For this review, use the dimensioned drawing (mm, ordinates from the lowest corner) and the shaded views. A direction names the side the tool comes from. Round coordinates to 2 decimals unless told otherwise and drop trailing zeros. Loops run counter-clockwise (first coordinate to the right, second up) from the corner with the lowest first, then second, coordinate; pieces in that order, holes last. Notation, with made-up numbers: M 4,55 L 48,55 A32 cw 48,91 Z; hole C 37,46.5 d7. An arc over 180 degrees is marked long. Answer as a JSON object with one key per item and string values. Group by question number.
Item 1: The part is to be moulded in two halves that separate along Z. For the marked faces 3, 4, 5 and 6, say which applies: +Z half, -Z half, draft (parallel to the pull), parting line (faces both ways), or undercut.
Item 2: To check wall thickness, follow line 1 (Y direction, x = 15, z = 20.3); line 2 (Y direction, x = 9.25, z = 21); line 3 (X direction, y = 13, z = 15). State the ranges of each line that lie inside material, in increasing order.
Item 3: Consider section C-C (x = 12). Give the boundary of the cut face in (y, z) (1 decimal).
Item 4: Consider section D-D (z = 20.5). Give the boundary of the cut face in (x, y) (1 decimal), and give its area (3 significant figures).
Item 5: Insertion check: P1, Ø3, axis at x = 15, y = 8, coming from the +Z side; P2, Ø12, axis at x = 18, y = 9.5, coming from the -Z side; P3, Ø4, axis at x = 18.5, y = 19.5, coming from the +Z side (1 decimal); P4, Ø6.5, axis at x = 15, z = 15, coming from the -Y side. Each pin has a flat end and moves straight along its axis. Give the tip position at first contact, or say it passes through.
Item 6: Consider section A-A (x = 15). Give the boundary of the cut face in (y, z) (1 decimal).
Item 7: Consider section B-B (z = 15). Give the boundary of the cut face in (x, y).
Item 8: Tool access review of the marked faces 1 and 2: name each direction out of +Z, -Z, +X, -X, +Y, -Y from which nothing blocks a thin tool from reaching the whole face with its end or side.
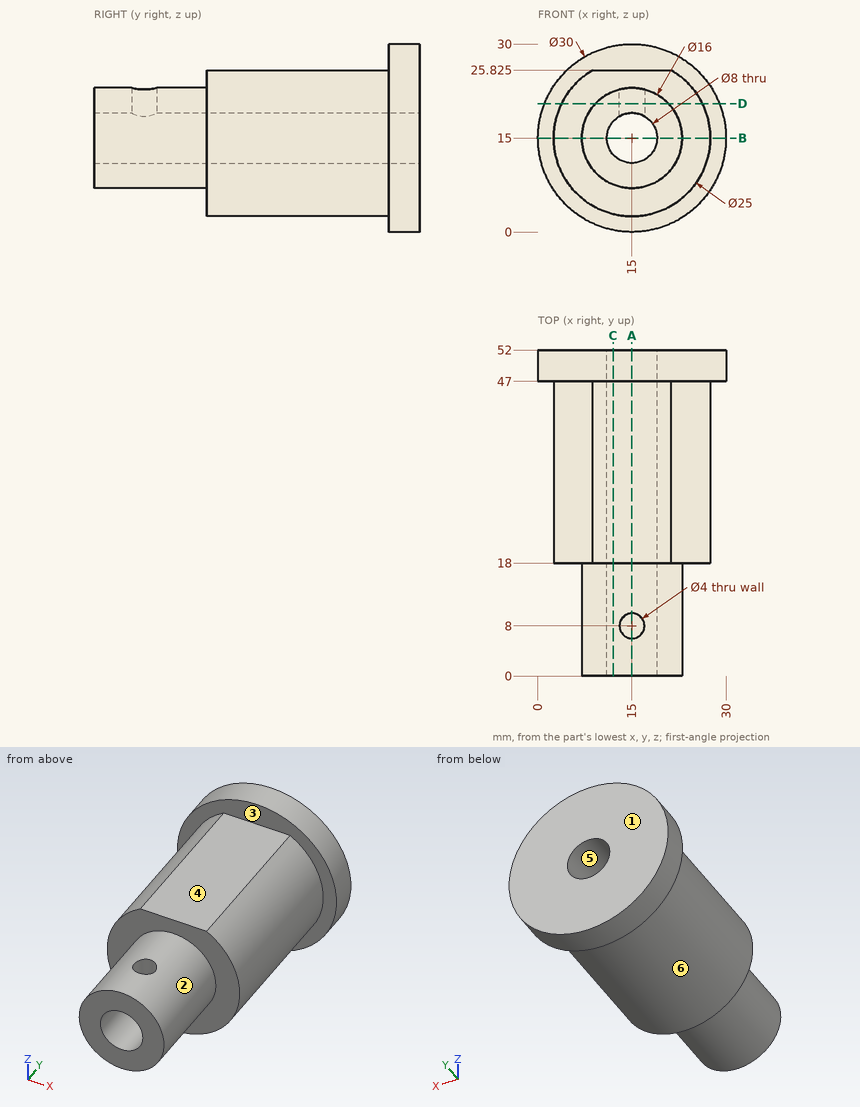
Geometry results:
{
 "1": {"face 3": "draft", "face 4": "+Z half", "face 5": "undercut", "face 6": "parting line"},
 "2": {"line 1": "y = 0 to 6, 10 to 52", "line 2": "y = 18 to 52", "line 3": "x = 7 to 11, 19 to 23"},
 "3": {"outline": "M 0,7.6 L 18,7.6 L 18,2.9 L 47,2.9 L 47,0.3 L 52,0.3 L 52,12.4 L 0,12.4 Z; M 0,17.6 L 52,17.6 L 52,29.7 L 47,29.7 L 47,25.8 L 18,25.8 L 18,22.4 L 0,22.4 Z"},
 "4": {"outline": "M 1,47 L 3.8,47 L 3.8,18 L 9.2,18 L 9.2,0 L 20.8,0 L 20.8,18 L 26.2,18 L 26.2,47 L 29,47 L 29,52 L 1,52 Z; hole C 15,8 d4", "area": "987 mm^2"},
 "5": {"P1": "stops at z = 11.29", "P2": "stops at z = 7", "P3": "stops at z = 25.8", "P4": "passes through"},
 "6": {"outline": "M 0,7 L 18,7 L 18,2.5 L 47,2.5 L 47,0 L 52,0 L 52,11 L 0,11 Z; M 0,19 L 6,19 L 6,23 L 0,23 Z; M 10,19 L 52,19 L 52,30 L 47,30 L 47,25.8 L 18,25.8 L 18,23 L 10,23 Z"},
 "7": {"outline": "M 0,47 L 2.5,47 L 2.5,18 L 7,18 L 7,0 L 11,0 L 11,52 L 0,52 Z; M 19,0 L 23,0 L 23,18 L 27.5,18 L 27.5,47 L 30,47 L 30,52 L 19,52 Z"},
 "8": {"face 1": "+Z, -Z, +X, -X, +Y", "face 2": "-Y"}
}
